Read the model definition and answer for the solid it produces. Units are mm, in the model's axes. Face numbers are marked on the shaded views. Coordinates: 2 decimals unless noted, no trailing zeros. Loops run counter-clockwise (first coordinate to the right, second up) from the corner with the lowest first, then second, coordinate; pieces in that order, holes last.
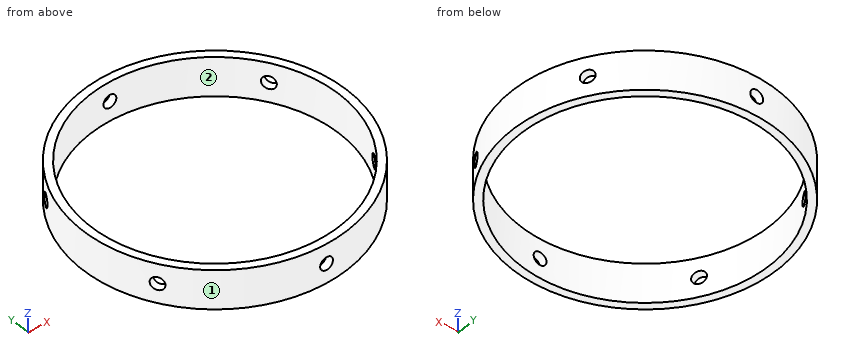
from build123d import *

# Parameters (mm, degrees)
SKETCH1_R           = 33.75
SKETCH1_R_2         = 31.75
BOSS_EXTRUDE1_DEPTH = 5
SKETCH3_W           = 1.65
SKETCH3_H           = 33.75
CIRPATTERN1_COUNT   = 6


with BuildPart() as part:
    # Sketch1 → Boss-Extrude1 (new, symmetric)
    with BuildSketch(Plane.XY):
        Circle(SKETCH1_R)
        Circle(SKETCH1_R_2, mode=Mode.SUBTRACT)
    extrude(amount=BOSS_EXTRUDE1_DEPTH, both=True)

    # Sketch3 → M4x0.7 Tapped Hole1 (revolve, cut)
    with BuildSketch(Plane(origin=(0, 0, 0), x_dir=(0, 0, -1), z_dir=(1, 0, 0))):
        with Locations((0.825, 16.875)):
            Rectangle(SKETCH3_W, SKETCH3_H)
    m4x0_7_tapped_hole1 = revolve(axis=Axis((0, -6.35, 0), (0, 1, 0)), mode=Mode.SUBTRACT)

    # CirPattern1: M4x0.7 Tapped Hole1 ×6 about axis
    cirpattern1_axis = Axis((0, 0, 5), (0, 0, -1))
    for i in range(1, CIRPATTERN1_COUNT):
        add(m4x0_7_tapped_hole1.rotate(cirpattern1_axis, i * 360 / CIRPATTERN1_COUNT), mode=Mode.SUBTRACT)


solid = part.part
Item 1: Given pin 1 (4 mm diameter, centred on x = 0, z = 0, fed in from +Y); pin 2 (3 mm diameter, centred on x = 0, z = 0, fed in from -Y); pin 3 (5 mm diameter, centred on y = 25, z = -4, fed in from +X); pin 4 (1 mm diameter, centred on y = 1.5, z = 0, fed in from +X), each flat-ended and moving along its own axis, determine where each tip first touches the part or whether it passes through.
Numbers:
pin 1: stops at y = 33.75
pin 2: passes through
pin 3: stops at x = 25.16
pin 4: stops at x = 33.74
Item 2: A cutting plane is placed at B-B on z = 0. Determine the outline of the cut face in (x, y), then the cut area to 3 significant figures.
Numbers:
outline: (-30.02, -15.43) - (-28.28, -14.42) arc R31.75 cw to (-28.28, 14.42) - (-30.02, 15.43) arc R33.75 ccw to start; (-28.37, -18.28) arc R33.75 ccw to (-1.65, -33.71) - (-1.65, -31.71) arc R31.75 cw to (-26.63, -17.28) - close; (-28.37, 18.28) - (-26.63, 17.28) arc R31.75 cw to (-1.65, 31.71) - (-1.65, 33.71) arc R33.75 ccw to start; (1.65, -33.71) arc R33.75 ccw to (28.37, -18.28) - (26.63, -17.28) arc R31.75 cw to (1.65, -31.71) - close; (1.65, 31.71) arc R31.75 cw to (26.63, 17.28) - (28.37, 18.28) arc R33.75 ccw to (1.65, 33.71) - close; (28.28, -14.42) - (30.02, -15.43) arc R33.75 ccw to (30.02, 15.43) - (28.28, 14.42) arc R31.75 cw to start
area: 372 mm2
Item 3: Determine the mould class of the marked faces 1 and 2 for opening direction X: released by +X, released by -X, zero draft, split by the parting line, or undercut.
Numbers:
face 1: split by the parting line
face 2: undercut
Item 4: Find the intervals of material crossed by line 1 along X through (y, z) = (1, -3); line 2 along Z through (x, y) = (0, 32); line 3 along Y through (x, z) = (-10, 4), in increasing order.
Numbers:
line 1: x = -33.74 to -31.73, 31.73 to 33.74
line 2: z = -5 to -1.65, 1.65 to 5
line 3: y = -32.23 to -30.13, 30.13 to 32.23
Item 5: A cutting plane is placed at C-C on x = -5.5. Determine the outline of the cut face in (y, z), then the cut area to 3 significant figures.
Numbers:
outline: (-33.3, -5) - (-31.27, -5) - (-31.27, 5) - (-33.3, 5) - close; (31.27, -5) - (33.3, -5) - (33.3, 5) - (31.27, 5) - close
area: 40.6 mm2
Item 6: A cutting plane is placed at A-A on y = 0. Determine the outline of the cut face in (x, z).
Numbers:
outline: (-33.75, -5) - (-31.75, -5) - (-31.75, 5) - (-33.75, 5) - close; (31.75, -5) - (33.75, -5) - (33.75, 5) - (31.75, 5) - close
